Job drawing, mm, ordinate dimensions from the low corner. One solid piece. A direction names the side the tool comes from. Give positions to 0.01 mm unless a question says otherwise; leave off trailing zeros. Loops run counter-clockwise (first coordinate to the right, second up) from the corner with the lowest first, then second, coordinate; pieces in that order, holes last.
Item 1: Saw through at B-B on x = 63.5. Give the cut face in (y, z).
Item 2: Saw through at A-A on z = 13. Give the cut face in (x, y).
Item 3: Saw through at C-C on y = 25. Give the cut face in (x, z), plus the area to 3 significant figures.
Item 4: Which spindle directions (+Z, -Z, +X, -X, +Y, -Y) get a long thin tool onto all of the face, cutting with end or side? Do the marked faces 4 and 5. Say none if no direction does.
Item 5: Saw through at D-D on x = 33. Give the cut face in (y, z).
Item 6: Drop flat-ended pins along their axis: P1, Ø10, axis at x = 132.5, y = 8, coming from the +Z side; P2, Ø2, axis at x = 49, y = 38, coming from the +Z side. Give the stop position or say it passes through.
Item 7: Mould opens along Y. For the marked faces 1, 2 and 3 say: released by +Y, released by -Y, zero draft, split by the parting line, or undercut.
Item 8: Probe probe 1 along Y at (x, z) = (121, 19.25); probe 2 along Z at (x, y) = (108, 25.5); probe 3 along Z at (x, y) = (25.4, 1.5) (1 decimal). List the from-to ranges inside material, lowest first.
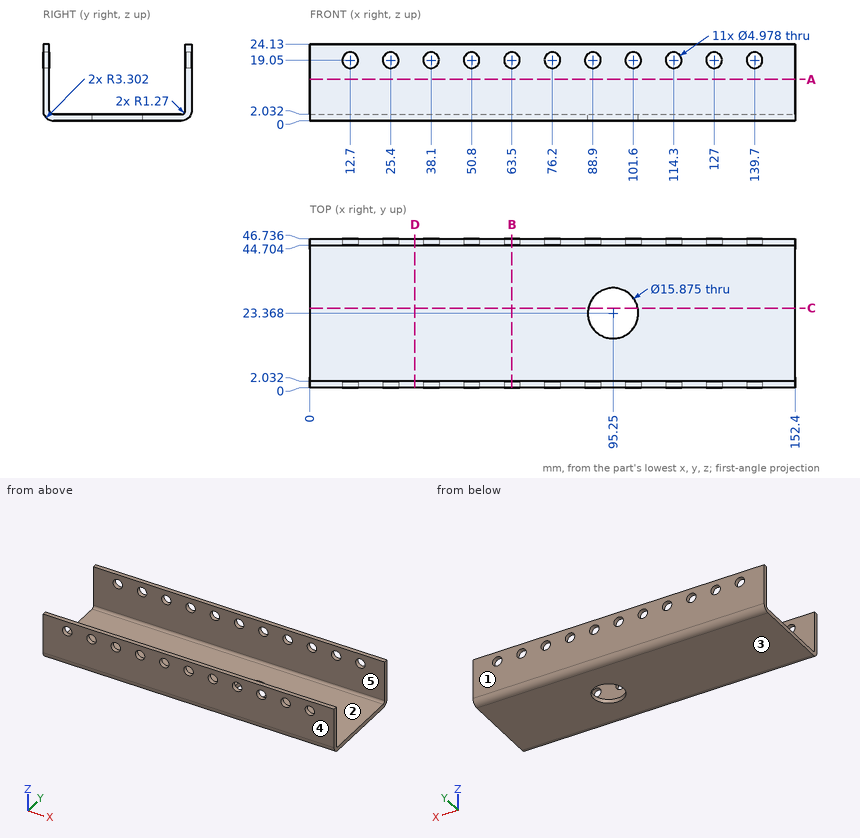
Results below:
1. outline: (0, 3.3) arc R3.3 ccw to (3.3, 0) - (43.43, 0) arc R3.3 ccw to (46.74, 3.3) - (46.74, 16.56) - (44.7, 16.56) - (44.7, 3.3) arc R1.27 cw to (43.43, 2.03) - (3.3, 2.03) arc R1.27 cw to (2.03, 3.3) - (2.03, 16.56) - (0, 16.56) - close; (0, 21.54) - (2.03, 21.54) - (2.03, 24.13) - (0, 24.13) - close; (44.7, 21.54) - (46.74, 21.54) - (46.74, 24.13) - (44.7, 24.13) - close
2. outline: (0, 0) - (152.4, 0) - (152.4, 2.03) - (0, 2.03) - close; (0, 44.7) - (152.4, 44.7) - (152.4, 46.74) - (0, 46.74) - close
3. outline: (0, 0) - (87.48, 0) - (87.48, 2.03) - (0, 2.03) - close; (103.02, 0) - (152.4, 0) - (152.4, 2.03) - (103.02, 2.03) - close
3. area: 278 mm2
4. face 4: +Z, -Z, +X, -X, -Y
4. face 5: +Z, +X, -X
5. outline: (0, 3.3) arc R3.3 ccw to (3.3, 0) - (43.43, 0) arc R3.3 ccw to (46.74, 3.3) - (46.74, 24.13) - (44.7, 24.13) - (44.7, 3.3) arc R1.27 cw to (43.43, 2.03) - (3.3, 2.03) arc R1.27 cw to (2.03, 3.3) - (2.03, 24.13) - (0, 24.13) - close
6. P1: stops at z = 2.07
6. P2: stops at z = 2.03
7. face 1: released by +Y
7. face 2: undercut
7. face 3: zero draft
8. probe 1: y = 0 to 2.03, 44.7 to 46.74
8. probe 2: z = 0 to 2.03
8. probe 3: z = 0.5 to 16.6, 21.5 to 24.1
